Build history of the part. All positions in model axes, mm. A direction names the side the tool comes from. Give positions to 0.01 mm unless a question says otherwise; leave off trailing zeros. Loops run counter-clockwise (first coordinate to the right, second up) from the corner with the lowest first, then second, coordinate; pieces in that order, holes last. Notation, with made-up numbers: M -26.5,45 L 26.5,45 A20 cw 26.5,57 Z; hole C 77.5,40 d3. An arc over 180 degrees is marked long. Answer in a Markdown table with one row per item. Add a question column.
```python
from build123d import *

# Parameters (mm, degrees)
SKETCH_1_W      = 2
SKETCH_1_H      = 30
EXTRUDE_3_DEPTH = 2
SKETCH_3_W      = 2
SKETCH_3_H      = 19.963569182
SKETCH_3_H_2    = 20
EXTRUDE_4_DEPTH = 12


with BuildPart() as part:
    # 草图1 → 凸台-拉伸3 (new body)
    with BuildSketch(Plane(origin=(0, 0, 0), x_dir=(1, 0, 0), z_dir=(0, 1, 0))):
        Polygon((100, 40), (0, 40), (0, 35), (0, 5), (0, 0), (38, 0), (38, 20), (40, 20), (40, 0), (60, 0), (60, 20), (62, 20), (62, 0), (100, 0), (100, 5), (100, 35), align=None)
        with Locations((-1, 20)):
            Rectangle(SKETCH_1_W, SKETCH_1_H)
        with Locations((101, 20)):
            Rectangle(SKETCH_1_W, SKETCH_1_H)
    extrude(amount=EXTRUDE_3_DEPTH)

    # 草图3 → 凸台-拉伸4 (add)
    with BuildSketch(Plane(origin=(0, 0, 0), x_dir=(1, 0, 0), z_dir=(0, 1, 0))):
        with Locations((39, 9.981784591)):
            Rectangle(SKETCH_3_W, SKETCH_3_H)
        with Locations((61, 10)):
            Rectangle(SKETCH_3_W, SKETCH_3_H_2)
    extrude(amount=EXTRUDE_4_DEPTH)


solid = part.part
```
(1) Slice it at B-B, the plane z = -12.5. Give the cut face in (x, y).
(2) Slice it at A-A, the plane y = 5.75. Give the cut face in (x, z).
(3) Wall check: line 1 (X direction, y = 8.25, z = -4); line 2 (Y direction, x = 35.5, z = -9.5). Give the ranges that are in metal, low to high.
(4) Tool access for faces 1 (the flat face through (0, 1, -3)), 2 (the flat face through (40, 7, -10)), 3 (the flat face through (100, 1, -37)): list every direction of +Z, -Z, +X, -X, +Y, -Y with a clear straight run to the whole face (end or side of a thin tool).
(5) Slice it at D-D, the plane z = -23. Give the cut face in (x, y), then the cut area to 3 significant figures.
(6) Slice it at C-C, the plane x = 94. Give the cut face in (y, z).
(7) Pin check, flat tips, straight feed: pin 1 (1 mm diameter, centred on y = 1, z = -3.5, fed in from +X); pin 2 (2 mm diameter, centred on x = 43.5, z = -21, fed in from -Y); pin 3 (1 mm diameter, centred on x = 101, y = 1, fed in from -Z); pin 4 (2 mm diameter, centred on x = 101.5, y = 0.5, fed in from +Z). Stop position of each tip, or through.
Solution:
| question | item | result |
|---|---|---|
| 1 | outline | M -2,0 L 102,0 L 102,2 L 62,2 L 62,12 L 60,12 L 60,2 L 40,2 L 40,12 L 38,12 L 38,2 L -2,2 Z |
| 2 | outline | M 38,-19.96 L 40,-19.96 L 40,0 L 38,0 Z; M 60,-20 L 62,-20 L 62,0 L 60,0 Z |
| 3 | line 1 | 38 to 40, 60 to 62 |
| 3 | line 2 | 0 to 2 |
| 4 | face 1 | +Z, -X, +Y, -Y |
| 4 | face 2 | +Z, -Z, +Y |
| 4 | face 3 | -Z, +X, +Y, -Y |
| 5 | outline | M -2,0 L 102,0 L 102,2 L -2,2 Z |
| 5 | area | 208 mm^2 |
| 6 | outline | M 0,-40 L 2,-40 L 2,0 L 0,0 Z |
| 7 | pin 1 | x = 100 |
| 7 | pin 2 | y = 0 |
| 7 | pin 3 | z = -35 |
| 7 | pin 4 | z = -5 |
